Here's how the part is built. I have some questions about the finished solid (model axes, mm). A direction names the side the tool comes from. Coordinates: 2 decimals unless noted, no trailing zeros. Write each loop counter-clockwise with the first axis right and the second up, starting at its lowest first coordinate (ties: lowest second). Pieces come first, ordered by that corner, then holes. Notation, with made-up numbers: M 72.25,0.25 L 96.25,0.25 A22 cw 96.25,34.25 Z; hole C 61,34.25 d2. An arc over 180 degrees is marked long. Use one line per item in the form item = value. Start each with the question number.
1. I want a section at D-D, the plane x = 5.5. List the corners of the cut face in (y, z) for me.
2. I'm going to push flat-ended pins straight in: pin 1 Ø2 at (x, y) = (18, -4.5) entering from -Z; pin 2 Ø0.8 at (y, z) = (3.5, 0.5) entering from -X; pin 3 Ø0.5 at (x, z) = (23, 0.5) entering from -Y. Where does each tip first touch, or does it pass through?
3. I want a section at B-B, the plane z = 0.25. List the corners of the cut face in (x, y) for me.
4. I want a section at A-A, the plane y = 0. List the corners of the cut face in (x, z) for me.
5. Please list where these lines run through material, in increasing order: line 1 along Y through (x, z) = (50, 0.55); line 2 along X through (y, z) = (3, 0.7); line 3 along Y through (x, z) = (37.5, 0.8). Write a range as [from, to].
6. Thinking about a two-plate mould opening in X: for faces 4 (the face through (11, 3.85, 1)), 5 (the face through (25, 2, 0)), which applies, released by +X, released by -X, zero draft, split by the parting line, or undercut?
7. I want a section at C-C, the plane x = 48.5. List the corners of the cut face in (y, z) for me.
8. On a 3-axis mill with a long thin cutter (end or side, diameter ignored), from which of +Z, -Z, +X, -X, +Y, -Y can I reach the whole of each face in a straight line? I mean faces 1 (the face through (36.1, 3, 1)), 2 (the face through (25, 2, 1.588)), 3 (the face through (25, -1.65, 1)). Say none if no direction works.
from build123d import *

# Parameters (mm, degrees)
SKETCH1_W           = 4.9
SKETCH1_H           = 1.5
SKETCH1_R           = 6.35
SKETCH1_W_2         = 3.125
SKETCH1_H_2         = 3.125
SKETCH1_R_2         = 2.25
BOSS_EXTRUDE1_DEPTH = 1.5875


with BuildPart() as part:
    # Sketch1 → Boss-Extrude1 (new body)
    # profile 1 of 3: a face of its own
    with BuildSketch(Plane.XY):
        with BuildLine():
            Line((50, 6.35), (0, 6.35))
            ThreePointArc((0, 6.35), (4.490128061, 4.490128061), (6.35, 0))
            ThreePointArc((6.35, 0), (6.295234812, -0.83217706), (6.131883887, -1.65))
            Line((6.131883887, -1.65), (43.868116113, -1.65))
            ThreePointArc((43.868116113, -1.65), (44.960158733, 3.862965182), (50, 6.35))
        make_face()
        with Locations((11.45, 3.1)):
            Rectangle(SKETCH1_W, SKETCH1_H, mode=Mode.SUBTRACT)
        with Locations((38.55, 3.1)):
            Rectangle(SKETCH1_W, SKETCH1_H, mode=Mode.SUBTRACT)
    # profile 2 of 3: a face of its own
    with BuildSketch(Plane.XY):
        Circle(SKETCH1_R)
        Rectangle(SKETCH1_W_2, SKETCH1_H_2, mode=Mode.SUBTRACT)
    # profile 3 of 3: a face of its own
    with BuildSketch(Plane.XY):
        with Locations((50, 0)):
            Circle(SKETCH1_R)
        with Locations((50, 0)):
            Circle(SKETCH1_R_2, mode=Mode.SUBTRACT)
    extrude(amount=BOSS_EXTRUDE1_DEPTH)


solid = part.part
Answer list:
q1.outline = M -3.17,0 L 6.35,0 L 6.35,1.59 L -3.17,1.59 Z
q2.pin_1 = through
q2.pin_2 = -5.54
q2.pin_3 = -1.65
q3.outline = M 0,6.35 A6.35 ccw long 6.13,-1.65 L 43.87,-1.65 A6.35 ccw long 50,6.35 Z; hole M -1.56,-1.56 L 1.56,-1.56 L 1.56,1.56 L -1.56,1.56 Z; hole M 9,2.35 L 13.9,2.35 L 13.9,3.85 L 9,3.85 Z; hole M 36.1,2.35 L 41,2.35 L 41,3.85 L 36.1,3.85 Z; hole C 50,0 d4.5
q4.outline = M -6.35,0 L -1.56,0 L -1.56,1.59 L -6.35,1.59 Z; M 1.56,0 L 47.75,0 L 47.75,1.59 L 1.56,1.59 Z; M 52.25,0 L 56.35,0 L 56.35,1.59 L 52.25,1.59 Z
q5.line_1 = [-6.35, -2.25], [2.25, 6.35]
q5.line_2 = [-5.6, 9], [13.9, 36.1], [41, 55.6]
q5.line_3 = [-1.65, 2.35], [3.85, 6.35]
q6.face_4 = undercut
q6.face_5 = zero draft
q7.outline = M -6.17,0 L -1.68,0 L -1.68,1.59 L -6.17,1.59 Z; M 1.68,0 L 6.35,0 L 6.35,1.59 L 1.68,1.59 Z
q8.face_1 = +Z, -Z
q8.face_2 = +Z, +X, -X, +Y, -Y
q8.face_3 = +Z, -Z, -Y
